```python
from build123d import *

# Parameters (mm, degrees)
F0_W         = 1.3692331631
F0_H         = 7.834737435
F0_W_2       = 6.5
F0_H_2       = 0.9
F0_W_3       = 0.6192331631
F0_H_3       = 1.05
F0_H_4       = 13.165262565
F0_W_4       = 0.8807668369
F0_W_5       = 1.6307668369
F1_DEPTH     = 0.9
F2_DEPTH     = 1.5
F3_DEPTH     = 7.8
F5_W         = 9.5
F5_H         = 19.2867757659
F6_DEPTH     = 1.5
F7_R         = 3
F8_DEPTH     = 20
F9_T1_DEPTH  = 5.3
F9_T3_DEPTH  = 5.5
F9_T5_DEPTH  = 22.2867757659
F9_T7_DEPTH  = 27
F9_S11_W     = 2
F9_S11_H     = 2
F9_T12_DEPTH = 2
F9_S17_W     = 2
F9_S17_H     = 2
F9_T18_DEPTH = 2
F9_S23_W     = 2
F9_S23_H     = 2
F9_T24_DEPTH = 2
F9_S29_W     = 2
F9_S29_H     = 2
F9_T30_DEPTH = 2
F10_R        = 2.7204865104
F11_DEPTH    = 6


# Not quite as in the source:
# - a fillet or chamfer that OpenCascade refuses, or shapes differently, is made with other operations: its cross-section is extruded or revolved along the edge and cut away or added
# - a feature names something its author has since deleted; it is built from what else it names


with BuildPart() as f1:
    # F0 (on Top) → F1 (new body)
    with BuildSketch(Plane.XY):
        Polygon((-4.75, 1.5), (-4.75, -1.5), (-3.3807668369, -1.5), (-3.3807668369, -0.45), (-4, -0.45), (-4, 0.45), (-3.3807668369, 0.45), (-3.3807668369, 1.5), align=None)
        Polygon((-3.3807668369, -0.45), (-3.3807668369, -1.5), (-3.1192331631, -1.5), (3.1192331631, -1.5), (3.1192331631, -0.45), align=None)
        with Locations((-4.0653834185, 5.4173687175)):
            Rectangle(F0_W, F0_H)
        with Locations((-0.1307668369, 0)):
            Rectangle(F0_W_2, F0_H_2)
        with Locations((-3.6903834185, 0)):
            Rectangle(F0_W_3, F0_H_2)
        with Locations((-0.1307668369, 5.4173687175)):
            Rectangle(F0_W_2, F0_H)
        with Locations((-0.1307668369, 0.975)):
            Rectangle(F0_W_2, F0_H_3)
        with Locations((-4.0653834185, 15.9173687175)):
            Rectangle(F0_W, F0_H_4)
        Polygon((3.1192331631, -0.45), (3.1192331631, -1.5), (3.3807668369, -1.5), (4.75, -1.5), (4.75, 1.5), (3.1192331631, 1.5), (3.1192331631, 0.45), (4, 0.45), (4, -0.45), align=None)
        with Locations((3.5596165815, 0)):
            Rectangle(F0_W_4, F0_H_2)
        with Locations((3.9346165815, 5.4173687175)):
            Rectangle(F0_W_5, F0_H)
        with Locations((-0.1307668369, 15.9173687175)):
            Rectangle(F0_W_2, F0_H_4)
        with Locations((3.9346165815, 15.9173687175)):
            Rectangle(F0_W_5, F0_H_4)
    extrude(amount=F1_DEPTH)

    # F0 (on Top) → F2 (join)
    with BuildSketch(Plane.XY):
        Polygon((-3.3807668369, -0.45), (-3.3807668369, -1.5), (-3.1192331631, -1.5), (3.1192331631, -1.5), (3.1192331631, -0.45), align=None)
        Polygon((3.1192331631, -0.45), (3.1192331631, -1.5), (3.3807668369, -1.5), (4.75, -1.5), (4.75, 1.5), (3.1192331631, 1.5), (3.1192331631, 0.45), (4, 0.45), (4, -0.45), align=None)
        Polygon((-4.75, 1.5), (-4.75, -1.5), (-3.3807668369, -1.5), (-3.3807668369, -0.45), (-4, -0.45), (-4, 0.45), (-3.3807668369, 0.45), (-3.3807668369, 1.5), align=None)
        with Locations((-0.1307668369, 0.975)):
            Rectangle(F0_W_2, F0_H_3)
        with Locations((-4.0653834185, 5.4173687175)):
            Rectangle(F0_W, F0_H)
        with Locations((3.9346165815, 5.4173687175)):
            Rectangle(F0_W_5, F0_H)
        with Locations((-0.1307668369, 5.4173687175)):
            Rectangle(F0_W_2, F0_H)
        with Locations((-4.0653834185, 15.9173687175)):
            Rectangle(F0_W, F0_H_4)
        with Locations((-0.1307668369, 15.9173687175)):
            Rectangle(F0_W_2, F0_H_4)
        with Locations((3.9346165815, 15.9173687175)):
            Rectangle(F0_W_5, F0_H_4)
    extrude(amount=F2_DEPTH)

    # F0 (on Top) → F3 (join)
    with BuildSketch(Plane.XY):
        Polygon((-4.75, 1.5), (-4.75, -1.5), (-3.3807668369, -1.5), (-3.3807668369, -0.45), (-4, -0.45), (-4, 0.45), (-3.3807668369, 0.45), (-3.3807668369, 1.5), align=None)
        Polygon((3.1192331631, -0.45), (3.1192331631, -1.5), (3.3807668369, -1.5), (4.75, -1.5), (4.75, 1.5), (3.1192331631, 1.5), (3.1192331631, 0.45), (4, 0.45), (4, -0.45), align=None)
        with Locations((-4.0653834185, 5.4173687175)):
            Rectangle(F0_W, F0_H)
        with Locations((3.9346165815, 5.4173687175)):
            Rectangle(F0_W_5, F0_H)
        with Locations((-4.0653834185, 15.9173687175)):
            Rectangle(F0_W, F0_H_4)
        with Locations((-0.1307668369, 15.9173687175)):
            Rectangle(F0_W_2, F0_H_4)
        with Locations((3.9346165815, 15.9173687175)):
            Rectangle(F0_W_5, F0_H_4)
    extrude(amount=F3_DEPTH)

    # F5 (on offset) → F6 (join)
    with BuildSketch(Plane.XY.offset(7.8)):
        with Locations((0, 12.856612117)):
            Rectangle(F5_W, F5_H)
    extrude(amount=F6_DEPTH)

    # F7 (on Front) → F8 (cut)
    with BuildSketch(Plane.XZ):
        with Locations((0, 4.5)):
            Circle(F7_R)
    extrude(amount=-F8_DEPTH, mode=Mode.SUBTRACT)

    # F9: fillet of radius 2 on 8 edges, made by hand

    # F9_s2 → F9_t1 (cut)
    with BuildSketch(Plane.XY.offset(2)):
        with BuildLine():
            ThreePointArc((4.75, 20.5), (4.1642135624, 21.9142135624), (2.75, 22.5))
            Line((2.75, 22.5), (4.75, 22.5))
            Line((4.75, 22.5), (4.75, 20.5))
        make_face()
        with BuildLine():
            ThreePointArc((-4.75, 20.5), (-4.1642135624, 21.9142135624), (-2.75, 22.5))
            Line((-2.75, 22.5), (-4.75, 22.5))
            Line((-4.75, 22.5), (-4.75, 20.5))
        make_face()
    extrude(amount=F9_T1_DEPTH, mode=Mode.SUBTRACT)

    # F9_s4 → F9_t3 (cut)
    with BuildSketch(Plane.YZ.offset(-2.75)):
        with BuildLine():
            ThreePointArc((20.5, 9.3), (21.9142135624, 8.7142135624), (22.5, 7.3))
            Line((22.5, 7.3), (22.5, 9.3))
            Line((22.5, 9.3), (20.5, 9.3))
        make_face()
        with BuildLine():
            ThreePointArc((20.5, 0), (21.9142135624, 0.5857864376), (22.5, 2))
            Line((22.5, 2), (22.5, 0))
            Line((22.5, 0), (20.5, 0))
        make_face()
    extrude(amount=F9_T3_DEPTH, mode=Mode.SUBTRACT)

    # F9_s6 → F9_t5 (cut)
    with BuildSketch(Plane.XZ.offset(-20.5)):
        with BuildLine():
            ThreePointArc((4.75, 7.3), (4.1642135624, 8.7142135624), (2.75, 9.3))
            Line((2.75, 9.3), (4.75, 9.3))
            Line((4.75, 9.3), (4.75, 7.3))
        make_face()
        with BuildLine():
            ThreePointArc((-4.75, 7.3), (-4.1642135624, 8.7142135624), (-2.75, 9.3))
            Line((-2.75, 9.3), (-4.75, 9.3))
            Line((-4.75, 9.3), (-4.75, 7.3))
        make_face()
    extrude(amount=F9_T5_DEPTH, mode=Mode.SUBTRACT)

    # F9_s8 → F9_t7 (cut)
    with BuildSketch(Plane.XZ.offset(-20.5)):
        with BuildLine():
            ThreePointArc((2.75, 0), (4.1642135624, 0.5857864376), (4.75, 2))
            Line((4.75, 2), (4.75, 0))
            Line((4.75, 0), (2.75, 0))
        make_face()
        with BuildLine():
            ThreePointArc((-4.75, 2), (-4.1642135624, 0.5857864376), (-2.75, 0))
            Line((-2.75, 0), (-4.75, 0))
            Line((-4.75, 0), (-4.75, 2))
        make_face()
    extrude(amount=F9_T7_DEPTH, mode=Mode.SUBTRACT)


with BuildPart() as f9_tool10:
    # F9_s11 → F9_t12 (new body)
    with BuildSketch(Plane.YZ.offset(2.75)):
        with Locations((21.5, 8.3)):
            Rectangle(F9_S11_W, F9_S11_H)
    extrude(amount=F9_T12_DEPTH)

    # F9_s13 → F9_t14 (revolve, cut)
    with BuildSketch(Plane(origin=(2.75, 20.5, 7.3), x_dir=(0, -0.7071067812, -0.7071067812), z_dir=(0, -0.7071067812, 0.7071067812))):
        with BuildLine():
            ThreePointArc((0, -2), (2, 0), (0, 2))
            Line((0, 2), (0, -2))
        make_face()
    revolve(axis=Axis((2.75, 20.5, 7.3), (1, 0, 0)), mode=Mode.SUBTRACT)


with BuildPart() as f1_1:
    add(f1.part)

    # F9_t9: cut F9_tool10
    add(f9_tool10.part, mode=Mode.SUBTRACT)


with BuildPart() as f9_tool16:
    # F9_s17 → F9_t18 (new body)
    with BuildSketch(Plane.XY.offset(2)):
        with Locations((3.75, 21.5)):
            Rectangle(F9_S17_W, F9_S17_H)
    extrude(amount=-F9_T18_DEPTH)

    # F9_s19 → F9_t20 (revolve, cut)
    with BuildSketch(Plane(origin=(2.75, 20.5, 2), x_dir=(-0.7071067812, -0.7071067812, 0), z_dir=(0.7071067812, -0.7071067812, 0))):
        with BuildLine():
            ThreePointArc((0, -2), (2, 0), (0, 2))
            Line((0, 2), (0, -2))
        make_face()
    revolve(axis=Axis((2.75, 20.5, 2), (0, 0, -1)), mode=Mode.SUBTRACT)


with BuildPart() as f1_2:
    add(f1_1.part)

    # F9_t15: cut F9_tool16
    add(f9_tool16.part, mode=Mode.SUBTRACT)


with BuildPart() as f9_tool22:
    # F9_s23 → F9_t24 (new body)
    with BuildSketch(Plane.YZ.offset(-2.75)):
        with Locations((21.5, 8.3)):
            Rectangle(F9_S23_W, F9_S23_H)
    extrude(amount=-F9_T24_DEPTH)

    # F9_s25 → F9_t26 (revolve, cut)
    with BuildSketch(Plane(origin=(-2.75, 20.5, 7.3), x_dir=(0, -0.7071067812, -0.7071067812), z_dir=(0, 0.7071067812, -0.7071067812))):
        with BuildLine():
            ThreePointArc((0, -2), (2, 0), (0, 2))
            Line((0, 2), (0, -2))
        make_face()
    revolve(axis=Axis((-2.75, 20.5, 7.3), (-1, 0, 0)), mode=Mode.SUBTRACT)


with BuildPart() as f1_3:
    add(f1_2.part)

    # F9_t21: cut F9_tool22
    add(f9_tool22.part, mode=Mode.SUBTRACT)


with BuildPart() as f9_tool28:
    # F9_s29 → F9_t30 (new body)
    with BuildSketch(Plane.YZ.offset(-2.75)):
        with Locations((21.5, 1)):
            Rectangle(F9_S29_W, F9_S29_H)
    extrude(amount=-F9_T30_DEPTH)

    # F9_s31 → F9_t32 (revolve, cut)
    with BuildSketch(Plane(origin=(-2.75, 20.5, 2), x_dir=(0, -0.7071067812, 0.7071067812), z_dir=(0, -0.7071067812, -0.7071067812))):
        with BuildLine():
            ThreePointArc((0, -2), (2, 0), (0, 2))
            Line((0, 2), (0, -2))
        make_face()
    revolve(axis=Axis((-2.75, 20.5, 2), (-1, 0, 0)), mode=Mode.SUBTRACT)


with BuildPart() as f1_4:
    add(f1_3.part)

    # F9_t27: cut F9_tool28
    add(f9_tool28.part, mode=Mode.SUBTRACT)

    # F10 (on Top) → F11 (cut)
    with BuildSketch(Plane.XY):
        with Locations((0, 17.4578037113)):
            Circle(F10_R)
    extrude(amount=F11_DEPTH, mode=Mode.SUBTRACT)


solid = f1_4.part
```
Source: CAD feature listing. Evaluate the final solid. Frame: model axes, mm. A direction names the side the tool comes from. Give positions to 0.01 mm unless a question says otherwise; leave off trailing zeros. Loops run counter-clockwise (first coordinate to the right, second up) from the corner with the lowest first, then second, coordinate; pieces in that order, holes last. Notation, with made-up numbers: (74.5, 13) - (83.5, 13) arc R20 ccw to (83.5, 46) - close; hole circle Ø2 at (-0.5, 84.5). An arc over 180 degrees is marked (long way). Use CSV: the item, a comma, the result in double quotes.
1) Mould query, pull axis X, two halves, no side actions, for faces 4 (the flat face through (3.119, -1, 5)), 5 (the flat face through (4, 1, 7.8)), 6 (the cylindrical face through (4.18, 21.9, 4.61)), 7 (the flat face through (-4, 0, 4)). Classes: +X half, -X half, draft (parallel to the pull), parting line (faces both ways), or undercut.
Worked out:
face 4,"undercut"
face 5,"draft"
face 6,"+X half"
face 7,"undercut"
2) Cut plane C-C (z = 1.25). Output: boundary loops of the cut face in (x, y), and give its area (3 significant figures).
Worked out:
outline,"(-4.6, -1.5) - (4.6, -1.5) - (4.6, 20.5) arc R1.85 ccw to (2.75, 22.35) - (-2.75, 22.35) arc R1.85 ccw to (-4.6, 20.5) - close; hole (-4, -0.45) - (4, -0.45) - (4, 0.45) - (-4, 0.45) - close; hole circle Ø5.44 at (0, 17.46)"
area,"188 mm^2"
3) Pin query (flat end, axial travel): P1, Ø1.5, axis at x = -1.5, z = 4.5, coming from the -Y side; P2, Ø1.2, axis at x = 2, z = 8.5, coming from the -Y side; P3, Ø1, axis at x = -4, y = 1, coming from the +Z side; P4, Ø3, axis at y = 17, z = 1.5, coming from the -X side. Return the tip coordinate at first contact, or that it passes through.
Worked out:
P1,"stops at y = 20"
P2,"stops at y = 3.21"
P3,"stops at z = 7.8"
P4,"stops at x = -4.75"
4) Set-up query: faces 1 (the flat face through (-3.381, -1, 5)), 2 (the flat face through (4, 0, 4)), 3 (the cylindrical face through (-0.354, 20.155, 1.625)). Return all of +Z, -Z, +X, -X, +Y, -Y with unobstructed straight access to the full face (end or side cutting, diameter ignored); none if empty.
Worked out:
face 1,"+Z, -Y"
face 2,"+Z"
face 3,"-Z"
5) Line query: line 1 (Z direction, x = 1.5, y = 6.25); line 2 (X direction, y = 17.5, z = 4.5); line 3 (X direction, y = 4, z = 6). Output: solid intervals per line, ascending.
Worked out:
line 1,"z = 0 to 1.5, 7.8 to 9.3"
line 2,"x = -4.75 to -3, 3 to 4.75"
line 3,"x = -4.75 to -3.38, 3.12 to 4.75"
6) Cut plane D-D (y = 13). Output: boundary loops of the cut face in (x, z).
Worked out:
outline,"(-4.75, 2) arc R2 ccw to (-2.75, 0) - (2.75, 0) arc R2 ccw to (4.75, 2) - (4.75, 7.3) arc R2 ccw to (2.75, 9.3) - (-2.75, 9.3) arc R2 ccw to (-4.75, 7.3) - close; hole circle Ø6 at (0, 4.5)"
7) Cut plane B-B (z = 4.5). Output: boundary loops of the cut face in (x, y).
Worked out:
outline,"(-4.75, -1.5) - (-3.38, -1.5) - (-3.38, -0.45) - (-4, -0.45) - (-4, 0.45) - (-3.38, 0.45) - (-3.38, 9.33) - (-3, 9.33) - (-3, 20) - (-0.97, 20) arc R2.72 cw to (0.97, 20) - (3, 20) - (3, 9.33) - (3.12, 9.33) - (3.12, 0.45) - (4, 0.45) - (4, -0.45) - (3.12, -0.45) - (3.12, -1.5) - (4.75, -1.5) - (4.75, 20.5) arc R2 ccw to (2.75, 22.5) - (-2.75, 22.5) arc R2 ccw to (-4.75, 20.5) - close"
8) Cut plane A-A (y = 4). Output: boundary loops of the cut face in (x, z), and give its area (3 significant figures).
Worked out:
outline,"(-4.75, 2) arc R2 ccw to (-2.75, 0) - (2.75, 0) arc R2 ccw to (4.75, 2) - (4.75, 7.3) arc R2 ccw to (2.75, 9.3) - (-2.75, 9.3) arc R2 ccw to (-4.75, 7.3) - close; hole (-3.38, 1.5) - (3.12, 1.5) - (3.12, 7.8) - (-3.38, 7.8) - close"
area,"44.0 mm^2"
